Read the model definition and answer for the solid it produces. Units are mm, in the model's axes. A direction names the side the tool comes from. Give positions to 0.01 mm unless a question says otherwise; leave off trailing zeros. Order: outer loops, then holes, each group sorted by start corner. A loop starts at its lowest first (then second) coordinate and runs counter-clockwise, first axis right, second up. Notation, with made-up numbers: (0, -14) - (31, -14) arc R19 ccw to (31, -6) - close; hole circle Ø1 at (70, 40.5). An arc over 180 degrees is marked (long way). Write item = value, one per line.
```python
from build123d import *


with BuildPart() as f1:
    # F0 (on Front) → F1 (revolve)
    with BuildSketch(Plane.XZ):
        with BuildLine():
            Line((0, 10), (0, 0))
            Line((0, 0), (3.5, 0))
            Line((3.5, 0), (6.5, 1))
            Line((6.5, 1), (9.5, 0))
            Line((9.5, 0), (11, 0))
            ThreePointArc((11, 0), (13.12132, 0.87868), (14, 3))
            Line((14, 3), (20, 3))
            Line((20, 3), (20, 4.083384))
            ThreePointArc((20, 4.083384), (20.585786, 5.497598), (22, 6.083384))
            Line((22, 6.083384), (36, 6.083384))
            ThreePointArc((36, 6.083384), (37.414214, 5.497598), (38, 4.083384))
            Line((38, 4.083384), (38, 3))
            Line((38, 3), (41, 3))
            Line((41, 3), (41, 2))
            Line((41, 2), (51, 2))
            ThreePointArc((51, 2), (53.12132, 2.87868), (54, 5))
            Line((54, 5), (54, 10))
            Line((54, 10), (41, 10))
            Line((41, 10), (38, 10))
            Line((38, 10), (20, 10))
            Line((20, 10), (14, 10))
            Line((14, 10), (9.5, 10))
            Line((9.5, 10), (6.5, 9))
            Line((6.5, 9), (3.5, 10))
            Line((3.5, 10), (0, 10))
        make_face()
    revolve(axis=Axis((26.417072, 0, 10), (1, 0, 0)))


solid = f1.part
```
1. Straight lines are drawn through the part: L1, parallel to X at y = -7, z = 4; L2, parallel to X at y = -6, z = 13.75; L3, parallel to Z at x = 3.5, y = -2.5. For each, find the intervals that lie inside material, in ascending order. Write a range as [from, to].
Recorded:
L1 = [0, 5.84], [7.16, 13.02]
L2 = [0, 14], [41, 53.17]
L3 = [0.32, 19.68]
2. Determine the mould class of faces 4 (the face through (6.354, -8.833, 11.962)), 5 (the face through (4.979, -0.189, 9.545)), 6 (the face through (41, -6, 14)) for opening direction Z: +Z half, -Z half, draft (parallel to the pull), parting line (faces both ways), or undercut.
Recorded:
face_4 = parting line
face_5 = undercut
face_6 = draft
3. Section C-C (x = 29.5) is taken. Determine the outline of the cut face in (y, z).
Recorded:
outline = circle Ø7.83 at (0, 10)
4. Flat-ended cylindrical pins translate along their axes: pin 1 (1 mm diameter, centred on y = 0, z = 17, fed in from +X); pin 2 (5 mm diameter, centred on x = 7, y = -7, fed in from +Z); pin 3 (4 mm diameter, centred on x = 25.5, y = 3.5, fed in from +Z). Find the tip coordinate at first contact, or state that the pin passes through.
Recorded:
pin_1 = 53.6
pin_2 = 18.28
pin_3 = 13.62
5. Section A-A (x = 39) is taken. Determine the outline of the cut face in (y, z), and give its area (3 significant figures).
Recorded:
outline = circle Ø14 at (0, 10)
area = 154 mm^2
6. For faces 1 (the face through (46.07, -7.81, 11.73)), 2 (the face through (17.042, -2.681, 3.534)), 3 (the face through (54, 0, 10)), determine the directions among +Z, -Z, +X, -X, +Y, -Y from which every point of the face is accessible in a straight line to the end or side of a thin tool.
Recorded:
face_1 = +X
face_2 = none
face_3 = +Z, -Z, +X, +Y, -Y
7. Section B-B (x = 4.5) is taken. Determine the outline of the cut face in (y, z).
Recorded:
outline = circle Ø19.33 at (0, 10); hole circle Ø0.67 at (0, 10)
